```python
from build123d import *

# Parameters (mm, degrees)
MODEL_W             = 97.14935
MODEL_H             = 129.19946
EXTRUDE_1_DEPTH     = 15
SKETCH_5_W          = 97.14935
SKETCH_5_H          = 129.19946
EXTRUDE_2_DEPTH     = 3
SKETCH_4_W          = 8
SKETCH_4_H          = 25
CUT_EXTRUDE_1_DEPTH = 2


with BuildPart() as part:
    # Model → 凸台-拉伸1 (new body)
    with BuildSketch(Plane.XY):
        with Locations((140.734852429, 91.461726055)):
            Rectangle(MODEL_W, MODEL_H)
        Polygon((102.160177429, 94.384872236), (102.160177429, 82.384872236), (102.160177429, 35.884872236), (102.160177429, 29.861996055), (179.309527429, 29.861996055), (179.309527429, 35.884872236), (179.309527429, 82.384872236), (179.309527429, 94.384872236), (179.309527429, 118.984602236), (179.309527429, 126.061456055), (179.309527429, 151.036037203), (102.185575181, 151.036037203), (102.160177429, 126.061456055), (102.160177429, 118.984602236), align=None, mode=Mode.SUBTRACT)
    extrude(amount=EXTRUDE_1_DEPTH)

    # 草图5 → 凸台-拉伸2 (add)
    with BuildSketch(Plane.XY.offset(15)):
        with Locations((140.734852429, 91.461726055)):
            Rectangle(SKETCH_5_W, SKETCH_5_H)
    extrude(amount=EXTRUDE_2_DEPTH)

    # 草图4 → 切除-拉伸1 (cut)
    with BuildSketch(Plane.XY):
        with Locations((98.160177429, 29.884872236)):
            Rectangle(SKETCH_4_W, SKETCH_4_H)
        with Locations((183.309527429, 88.384872236)):
            Rectangle(SKETCH_4_W, SKETCH_4_H)
        with Locations((98.160177429, 88.384872236)):
            Rectangle(SKETCH_4_W, SKETCH_4_H)
        with Locations((183.309527429, 29.884872236)):
            Rectangle(SKETCH_4_W, SKETCH_4_H)
    extrude(amount=CUT_EXTRUDE_1_DEPTH, mode=Mode.SUBTRACT)


solid = part.part
```
Design review of the part built by this model. Coordinates are the model's own, in mm. A direction names the side the tool comes from. Give positions to 0.01 mm unless a question says otherwise; leave off trailing zeros. Write each loop counter-clockwise with the first axis right and the second up, starting at its lowest first coordinate (ties: lowest second). Pieces come first, ordered by that corner, then holes.
(1) Add section D-D (y = 60). Give the boundary of the cut face in (x, z).
Checked values:
outline: (92.16, 0) - (102.16, 0) - (102.16, 15) - (179.31, 15) - (179.31, 0) - (189.31, 0) - (189.31, 18) - (92.16, 18) - close
(2) Add section B-B (y = 98.5). Give the boundary of the cut face in (x, z).
Checked values:
outline: (92.16, 0) - (94.16, 0) - (94.16, 2) - (102.16, 2) - (102.16, 15) - (179.31, 15) - (179.31, 2) - (187.31, 2) - (187.31, 0) - (189.31, 0) - (189.31, 18) - (92.16, 18) - close
(3) Wall thickness on line 1 along X through (y, z) = (90.5, 8); line 2 along Y through (x, z) = (138, 14); line 3 along Z through (x, y) = (165.5, 55): over which ranges is each line inside the solid? List them lowest first.
Checked values:
line 1: x = 92.16 to 102.16, 179.31 to 189.31
line 2: y = 26.86 to 29.86, 151.04 to 156.06
line 3: z = 15 to 18
(4) Tool access review of faces 5 (the face through (141, 151.036, 7)), 6 (the face through (140, 92, 18)), 7 (the face through (183, 35, 2)): name each direction out of +Z, -Z, +X, -X, +Y, -Y from which nothing blocks a thin tool from reaching the whole face with its end or side.
Checked values:
face 5: -Z
face 6: +Z, +X, -X, +Y, -Y
face 7: -Z, -Y
(5) Add section A-A (z = 8). Give the boundary of the cut face in (x, y).
Checked values:
outline: (92.16, 26.86) - (189.31, 26.86) - (189.31, 156.06) - (92.16, 156.06) - close; hole (102.16, 29.86) - (179.31, 29.86) - (179.31, 151.04) - (102.19, 151.04) - (102.16, 126.06) - close
(6) Clearance check with flat-ended pins moving along their axes: pin 1 Ø2.5 at (x, y) = (99, 31) entering from -Z; pin 2 Ø4 at (x, y) = (112.5, 130.5) entering from -Z; pin 3 Ø0.6 at (x, z) = (98, 1) entering from -Y. State where each tip first meets the part, or that it passes through.
Checked values:
pin 1: stops at z = 2
pin 2: stops at z = 15
pin 3: stops at y = 42.38
(7) Add section C-C (x = 129). Give the boundary of the cut face in (y, z).
Checked values:
outline: (26.86, 0) - (29.86, 0) - (29.86, 15) - (151.04, 15) - (151.04, 0) - (156.06, 0) - (156.06, 18) - (26.86, 18) - close
(8) Mouldability with a two-part tool opening along Y and no side actions: class faces 1 (the face through (140, 26.862, 9)), 2 (the face through (92.16, 91, 9)), 3 (the face through (179.31, 91, 7)), 4 (the face through (140, 156.061, 9)) as +Y half, -Y half, draft (parallel to the pull), parting line (faces both ways), or undercut.
Checked values:
face 1: -Y half
face 2: draft
face 3: undercut
face 4: +Y half
